Work out the finished part from the listing and answer in its coordinate system (mm). A direction names the side the tool comes from. Round coordinates to 2 decimals unless told otherwise and drop trailing zeros. Loops run counter-clockwise (first coordinate to the right, second up) from the corner with the lowest first, then second, coordinate; pieces in that order, holes last.
from build123d import *

# Parameters (mm, degrees)
CYLINDER_R     = 2
CYLINDER_DEPTH = 11
BOX_W          = 175
BOX_H          = 72
BOX_DEPTH      = 36
BOX002_W       = 7
BOX002_H       = 4
BOX002_DEPTH   = 10
BOX003_W       = 10
BOX003_H       = 33
BOX003_DEPTH   = 24


with BuildPart() as f_24v_cable:
    # Cylinder → Cylinder (new body)
    with BuildSketch(Plane(origin=(-7, 36, 18), x_dir=(0, 0, -1), z_dir=(1, 0, 0))):
        Circle(CYLINDER_R)
    extrude(amount=CYLINDER_DEPTH)


with BuildPart() as obj1:
    # Box → Box (new body)
    with BuildSketch(Plane.XY):
        with Locations((87.5, 36)):
            Rectangle(BOX_W, BOX_H)
    extrude(amount=BOX_DEPTH)


with BuildPart() as led:
    # Box002 → Box002 (new body)
    with BuildSketch(Plane(origin=(5, 18, 26), x_dir=(1, 0, 0), z_dir=(0, 0, 1))):
        with Locations((3.5, 2)):
            Rectangle(BOX002_W, BOX002_H)
    extrude(amount=BOX002_DEPTH)


with BuildPart() as fusion:
    # Box003 → Box003 (new body)
    with BuildSketch(Plane(origin=(167, 20, 6), x_dir=(1, 0, 0), z_dir=(0, 0, 1))):
        with Locations((5, 16.5)):
            Rectangle(BOX003_W, BOX003_H)
    extrude(amount=BOX003_DEPTH)

    # Fusion: union 24V Cable, obj1, LED
    add(f_24v_cable.part)
    add(obj1.part)
    add(led.part)


solid = fusion.part
Item 1: Section C-C, the plane z = 8 is taken. Give the vertices of the cut face in (x, y), plus the area to 3 significant figures.
Item 2: For faces 1 (the face through (-4, 34, 18)), 2 (the face through (-7, 36, 18)), determine the directions among +Z, -Z, +X, -X, +Y, -Y from which every point of the face is accessible in a straight line to the end or side of a thin tool.
Item 3: Section D-D, the plane y = 57.5 is taken. Give the vertices of the cut face in (x, z).
Item 4: Straight lines are drawn through the part: line 1 (X direction, y = 5, z = 11); line 2 (X direction, y = 34, z = 11.5). For each, find the intervals that lie inside material, in ascending order.
Item 5: Section B-B, the plane z = 18 is taken. Give the vertices of the cut face in (x, y), plus the area to 3 significant figures.
Item 6: Each of these flat-tipped pins is pushed along its axis until it touches: P1, Ø1.5, axis at x = 13.5, z = 18.5, coming from the -Y side; P2, Ø1.6, axis at x = 176.5, y = 39, coming from the +Z side; P3, Ø18, axis at y = 18.5, z = 11, coming from the -X side; P4, Ø1.5, axis at y = 64.5, z = 28.5, coming from the +X side. Where does it stop, or does it pass through?
Item 7: Section A-A, the plane y = 36 is taken. Give the vertices of the cut face in (x, z), plus the area to 3 significant figures.
Answer below:
1. outline: (0, 0) - (175, 0) - (175, 20) - (177, 20) - (177, 53) - (175, 53) - (175, 72) - (0, 72) - close
1. area: 12,700 mm2
2. face 1: -X
2. face 2: +Z, -Z, -X, +Y, -Y
3. outline: (0, 0) - (175, 0) - (175, 36) - (0, 36) - close
4. line 1: x = 0 to 175
4. line 2: x = 0 to 177
5. outline: (-7, 34) - (0, 34) - (0, 0) - (175, 0) - (175, 20) - (177, 20) - (177, 53) - (175, 53) - (175, 72) - (0, 72) - (0, 38) - (-7, 38) - close
5. area: 12,700 mm2
6. P1: stops at y = 0
6. P2: stops at z = 30
6. P3: stops at x = 0
6. P4: stops at x = 175
7. outline: (-7, 16) - (0, 16) - (0, 0) - (175, 0) - (175, 6) - (177, 6) - (177, 30) - (175, 30) - (175, 36) - (0, 36) - (0, 20) - (-7, 20) - close
7. area: 6,380 mm2
